Build history of the part. All positions in model axes, mm. A direction names the side the tool comes from. Round coordinates to 2 decimals unless told otherwise and drop trailing zeros. Order: outer loops, then holes, each group sorted by start corner. A loop starts at its lowest first (then second) coordinate and runs counter-clockwise, first axis right, second up. Notation, with made-up numbers: M 66.5,-0.75 L 109.5,-0.75 A29 cw 109.5,33.25 Z; hole C 88,-4 d6. An arc over 180 degrees is marked long. One line per item, written item: value. Start each with the question number.
Item 1: Two-plate mould, pull along Y, no slides. Class faces 5 (the cylindrical face through (19.584, 2.703, 0.07)), 6 (the cylindrical face through (-20, 0, 0)), 7 (the flat face through (-2.031, -32, 0)), 8 (the cylindrical face through (-34.992, -0.741, -0.014)): +Y half, -Y half, draft (parallel to the pull), parting line (faces both ways), or undercut.
Item 2: Band-saw the part on B-B, the plane x = 0. Write the cut outline in (y, z).
Item 3: Probe L1, parallel to X at y = 5.5, z = 2.75; L2, parallel to Y at x = 11, z = 2.5; L3, parallel to Y at x = -11, z = 0.25. List the from-to ranges inside material, lowest first.
Item 4: Band-saw the part on A-A, the plane y = 0. Write the cut outline in (x, z), then the cut area to 3 significant figures.
Item 5: Band-saw the part on C-C, the plane x = -11. Write the cut outline in (y, z).
Item 6: Pin check, flat tips, straight feed: pin 1 (2 mm diameter, centred on y = 5.5, z = 3, fed in from -X); pin 2 (2 mm diameter, centred on x = -23.5, y = 15.5, fed in from +Z); pin 3 (1.6 mm diameter, centred on x = -0.5, z = -0.5, fed in from -Y). Stop position of each tip, or through.
Item 7: Tool access for faces 1 (the flat face through (0, 29, 0)), 2 (the flat face through (1.969, -32, 0)), 3 (the cylindrical face through (-5.5, -24.9, 3)), 4 (the cylindrical face through (-5.5, -24.9, -3)): list every direction of +Z, -Z, +X, -X, +Y, -Y with a clear straight run to the whole face (end or side of a thin tool).
Item 8: Band-saw the part on D-D, the plane y = 31. Write the cut outline in (x, z).
Autodesk Inventor part; units mm, degrees
ref_plane "YZ Plane" through (0, 0, 0) normal (1, 0, 0) x (0, 1, 0)
ref_plane "XZ Plane" through (0, 0, 0) normal (0, 1, 0) x (-1, 0, 0)
ref_plane "XY Plane" through (0, 0, 0) normal (0, 0, 1) x (1, 0, 0)
sketch "Эскиз1" plane through (0, 0, 0) normal (0, 0, 1) x (1, 0, 0)
  circle A0 centre (0, 0) radius 35
  circle A1 centre (0, 0) radius 25.5
  circle A2 centre (11, 0) radius 9
  circle A3 centre (-11, 0) radius 9
  line L0 (-2.0313, 35) -> (1.9687, 35)
  line L1 (1.9687, 35) -> (1.9687, 29)
  line L2 (1.9687, 29) -> (-2.0313, 29)
  line L3 (-2.0313, 29) -> (-2.0313, 35)
  line L4 (-2.0313, -29) -> (1.9687, -29)
  line L5 (1.9687, -29) -> (1.9687, -35)
  line L6 (1.9687, -35) -> (-2.0313, -35)
  line L7 (-2.0313, -35) -> (-2.0313, -29)
  line L8 (-0.0313, 25.5) -> (-0.0313, -25.5)
  line L9 (-0.0313, -25.5) -> (-0.0313, -35)
  line L10 (-0.0313, 35) -> (-0.0313, 25.5)
  point P0 (-2.0313, 25.419)
  point P1 (-2.0313, -25.419)
  point P2 (1.9687, -25.4239)
  point P3 (1.9687, 25.4239)
  point P4 (1.9687, -34.9446)
  point P5 (1.9687, 34.9446)
  point P6 (-2.0313, 34.941)
  point P7 (-2.0313, -34.941)
  dimension "d0" = 70
  dimension "d1" = 51
  dimension "d2" = 18
  dimension "d3" = 18
  dimension "d4" = 11
  dimension "d5" = 11
  dimension "d6" = 40
  dimension "d7" = 4
  dimension "d8" = 4
  dimension "d9" = 6
  dimension "d10" = 6
  dimension "d11" = 2
  dimension "d12" = 2
  dimension "d17" = 0
  dimension "d18" = 0
extrude "Выдавливание1" add sketch "Эскиз1" along normal mid plane 10 contours L8 A1 | A1 L8
extrude "Выдавливание2" add sketch "Эскиз1" along normal mid plane 2 contours A0 L5 L4 L9 A1 L10 L2 L1 | L3 L2 L10 A1 L9 L4 L7 A0
equation "\"d0\" = dOuter"
equation "\"d1\" = dMount"
equation "\"d2\" = dHoles"
equation "\"d3\" = dHoles"
equation "\"d7\" = slotWidth"
equation "\"d8\" = slotWidth"
equation "\"d9\" = slotDepth"
equation "\"d10\" = slotDepth"
equation "\"d11\" = 0.5 * slotWidth"
equation "\"d12\" = 0.5 * slotWidth"
equation "\"dOuter\" = 70"
equation "\"dHoles\" = 18"
equation "\"hFlange\" = 4"
equation "\"hMount\" = 8"
equation "\"mountAngle\" = 60deg"
equation "\"dInternal\" = 44"
equation "\"dMount\" = 51"
equation "\"r2holes\" = 11"
equation "\"slotWidth\" = 4"
equation "\"slotDepth\" = 6"
properties part number "Spacer"
Output:
1. face 5: undercut
1. face 6: undercut
1. face 7: draft
1. face 8: parting line
2. outline: M -29,-1 L -25.5,-1 L -25.5,-5 L 25.5,-5 L 25.5,-1 L 29,-1 L 29,1 L 25.5,1 L 25.5,5 L -25.5,5 L -25.5,1 L -29,1 Z
3. L1: x = -24.9 to -18.12, -3.88 to 3.88, 18.12 to 24.9
3. L2: y = -23.01 to -9, 9 to 23.01
3. L3: y = -33.23 to -9, 9 to 33.23
4. outline: M -35,-1 L -25.5,-1 L -25.5,-5 L -20,-5 L -20,5 L -25.5,5 L -25.5,1 L -35,1 Z; M -2,-5 L 2,-5 L 2,5 L -2,5 Z; M 20,-5 L 25.5,-5 L 25.5,-1 L 35,-1 L 35,1 L 25.5,1 L 25.5,5 L 20,5 Z
4. area: 188 mm²
5. outline: M -33.23,-1 L -23.01,-1 L -23.01,-5 L -9,-5 L -9,5 L -23.01,5 L -23.01,1 L -33.23,1 Z; M 9,-5 L 23.01,-5 L 23.01,-1 L 33.23,-1 L 33.23,1 L 23.01,1 L 23.01,5 L 9,5 Z
6. pin 1: stops at x = -25.1
6. pin 2: stops at z = 1
6. pin 3: stops at y = -29
7. face 1: +Z, -Z, +Y
7. face 2: +Z, -Z, -Y
7. face 3: +Z
7. face 4: -Z
8. outline: M -16.25,-1 L -2.03,-1 L -2.03,1 L -16.25,1 Z; M 1.97,-1 L 16.25,-1 L 16.25,1 L 1.97,1 Z
